```python
from build123d import *

# Parameters (mm, degrees)
BOX001_W     = 12.7
BOX001_H     = 63.5
BOX001_DEPTH = 12.7
BOX002_W     = 76.2
BOX002_H     = 12.7
BOX002_DEPTH = 12.7


with BuildPart() as cube:
    # Box001 → Box001 (new body)
    with BuildSketch(Plane.XY.offset(406.4)):
        with Locations((6.35, 31.75)):
            Rectangle(BOX001_W, BOX001_H)
    extrude(amount=BOX001_DEPTH)


with BuildPart() as fusion:
    # Box002 → Box002 (new body)
    with BuildSketch(Plane(origin=(-31.75, -12.7, 406.4), x_dir=(1, 0, 0), z_dir=(0, 0, 1))):
        with Locations((38.1, 6.35)):
            Rectangle(BOX002_W, BOX002_H)
    extrude(amount=BOX002_DEPTH)

    # Fusion: union Cube
    add(cube.part)


solid = fusion.part
```
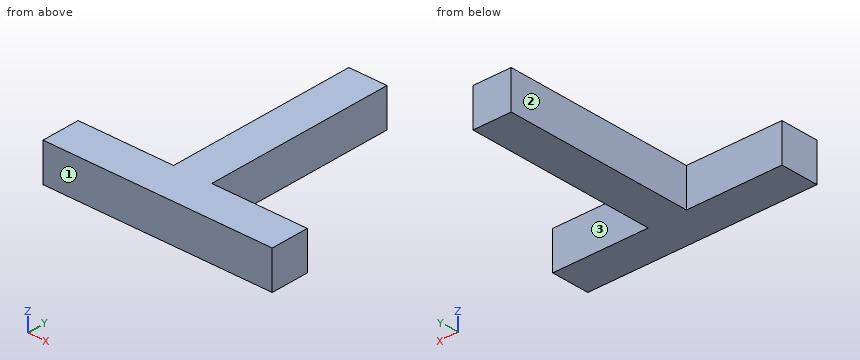
Check sheet for the modelled part. Datum: model origin and axes. Units: mm. Face numbers are marked on the shaded views. A direction names the side the tool comes from. Round coordinates to 2 decimals unless told otherwise and drop trailing zeros. Write each loop counter-clockwise with the first axis right and the second up, starting at its lowest first coordinate (ties: lowest second). Pieces come first, ordered by that corner, then holes. Notation, with made-up numbers: M 53.25,-12 L 64.25,-12 A15 ccw 64.25,6 Z; hole C -8,69 d8. An arc over 180 degrees is marked long. Write item = value, one per line. Start each with the question number.
1. Section check B-B, the plane y = 17. Record the cut outline in (x, z), then the cut area to 3 significant figures.
2. Section check C-C, the plane x = -3. Record the cut outline in (y, z), then the cut area to 3 significant figures.
3. Scan lines: line 1 (X direction, y = 2.5, z = 413.5); line 2 (Y direction, x = 38.5, z = 411.75). Record each from-to range of solid material in increasing order. Write a range as [from, to].
4. Gauge pin test, flat ends, axial feed: pin 1 (5 mm diameter, centred on x = 27, z = 411, fed in from +Y); pin 2 (4 mm diameter, centred on y = 24.5, z = 415.5, fed in from -X). Record the tip position at first contact, or that the pin passes through.
5. Tool access check on the marked faces 1, 2 and 3. Record the directions out of +Z, -Z, +X, -X, +Y, -Y that give a thin tool (end or side, any length) a straight path to the whole face; none if there is none.
6. Section check A-A, the plane z = 409.75. Record the cut outline in (x, y), then the cut area to 3 significant figures.
Results found:
q1.outline = M 0,406.4 L 12.7,406.4 L 12.7,419.1 L 0,419.1 Z
q1.area = 161 mm^2
q2.outline = M -12.7,406.4 L 0,406.4 L 0,419.1 L -12.7,419.1 Z
q2.area = 161 mm^2
q3.line_1 = [0, 12.7]
q3.line_2 = [-12.7, 0]
q4.pin_1 = 0
q4.pin_2 = 0
q5.face_1 = +Z, -Z, +X, -X, -Y
q5.face_2 = +Z, -Z, -X, +Y
q5.face_3 = +Z, -Z, +X, +Y
q6.outline = M -31.75,-12.7 L 44.45,-12.7 L 44.45,0 L 12.7,0 L 12.7,63.5 L 0,63.5 L 0,0 L -31.75,0 Z
q6.area = 1,770 mm^2
